The figure shows three views and two pictorial views of one solid part (mm, origin at its lowest corner). Answer the questions. Give positions to 0.01 mm unless a question says otherwise; leave off trailing zeros. Order: outer loops, then holes, each group sorted by start corner. A loop starts at its lowest first (then second) coordinate and runs counter-clockwise, first axis right, second up. Notation, with made-up numbers: M 58,16 L 78,16 A22 cw 78,51 Z; hole C 49.5,-26.5 d10. An arc over 180 degrees is marked long. One line per item, written item: value. Start each with the question number.
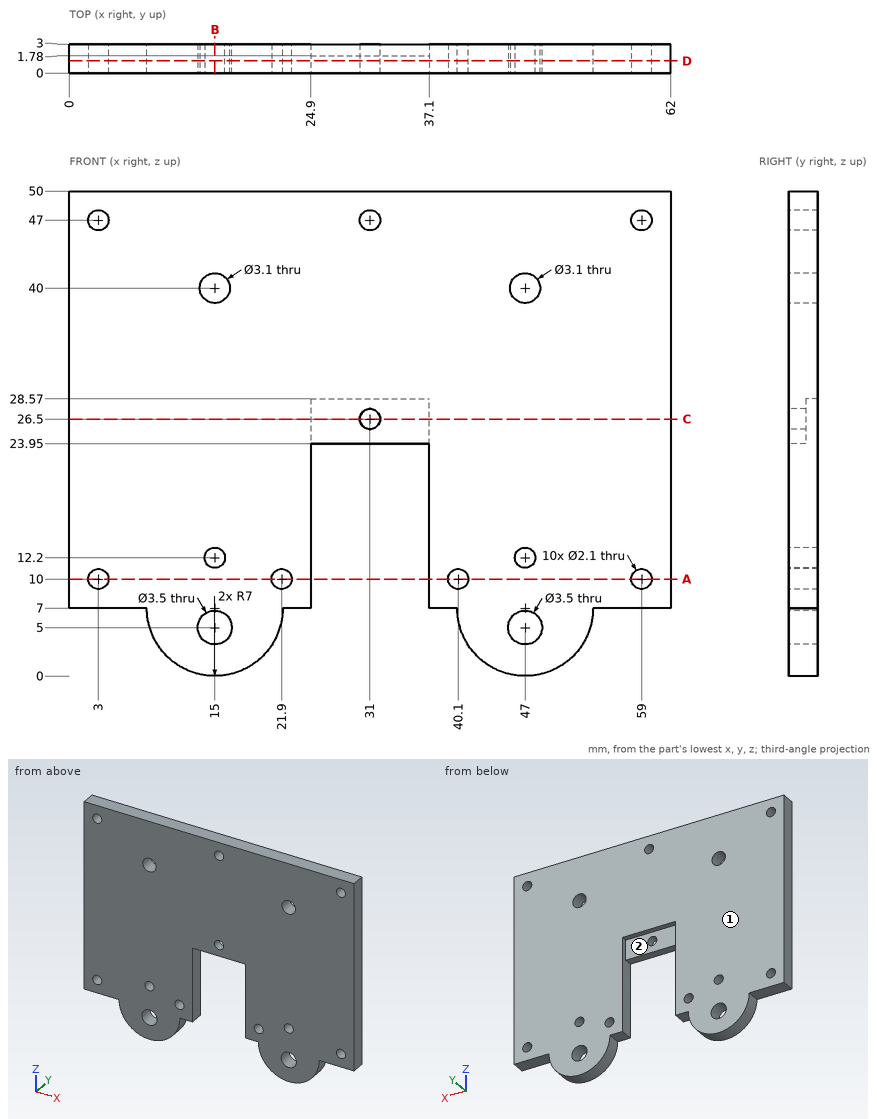
Q1. Find section A-A, the plane z = 10. Give the vertices of the cut face in (x, y), then the cut area to 3 significant figures.
Q2. Each of these flat-tipped pins is pushed along its axis until it touches: pin 1 (2.5 mm diameter, centred on x = 47, z = 12.2, fed in from -Y); pin 2 (1.3 mm diameter, centred on x = 21.9, z = 10, fed in from -Y); pin 3 (3 mm diameter, centred on x = 31, z = 24, fed in from +Y). Where does it stop, or does it pass through?
Q3. Consider probe 1 along X at (y, z) = (1.75, 40); probe 2 along X at (y, z) = (1.45, 47); probe 3 along X at (y, z) = (2.15, 26.5). Determine where each line is inside the solid, lowest interval first.
Q4. Find section B-B, the plane x = 15. Give the vertices of the cut face in (y, z), then the cut area to 3 significant figures.
Q5. Find section D-D, the plane y = 1.25. State how many separate pieces and enclosed holes the cut face has, then the cut area to 3 significant figures.
Q6. Determine the mould class of the marked faces 1 and 2 for opening direction X: released by +X, released by -X, zero draft, split by the parting line, or undercut.
Q7. Find section C-C, the plane z = 26.5. Give the vertices of the cut face in (x, y).
Evaluation:
1. outline: M 0,0 L 1.95,0 L 1.95,3 L 0,3 Z; M 4.05,0 L 20.85,0 L 20.85,3 L 4.05,3 Z; M 22.95,0 L 24.9,0 L 24.9,3 L 22.95,3 Z; M 37.1,0 L 39.05,0 L 39.05,3 L 37.1,3 Z; M 41.15,0 L 57.95,0 L 57.95,3 L 41.15,3 Z; M 60.05,0 L 62,0 L 62,3 L 60.05,3 Z
1. area: 124 mm2
2. pin 1: y = 0
2. pin 2: through
2. pin 3: y = 1.78
3. probe 1: 0 to 13.45, 16.55 to 45.45, 48.55 to 62
3. probe 2: 0 to 1.95, 4.05 to 29.95, 32.05 to 57.95, 60.05 to 62
3. probe 3: 0 to 24.9, 37.1 to 62
4. outline: M 0,0 L 3,0 L 3,3.25 L 0,3.25 Z; M 0,6.75 L 3,6.75 L 3,11.15 L 0,11.15 Z; M 0,13.25 L 3,13.25 L 3,38.45 L 0,38.45 Z; M 0,41.55 L 3,41.55 L 3,50 L 0,50 Z
4. area: 124 mm2
5. separate pieces: 1
5. enclosed holes: 14
5. area: 2,540 mm2
6. face 1: zero draft
6. face 2: undercut
7. outline: M 0,0 L 29.95,0 L 29.95,1.78 L 24.9,1.78 L 24.9,3 L 0,3 Z; M 32.05,0 L 62,0 L 62,3 L 37.1,3 L 37.1,1.78 L 32.05,1.78 Z
